For this review, take the finished solid that the model builds, in its own axes (mm). Coordinates: 2 decimals unless noted, no trailing zeros. Write each loop counter-clockwise with the first axis right and the second up, starting at its lowest first coordinate (ties: lowest second). Pieces come first, ordered by that corner, then holes.
```python
from build123d import *

# Parameters (mm, degrees)
F0_W     = 170
F0_H     = 40
F1_DEPTH = 1000
F3_DEPTH = 170.001
F4_SIZE2 = 25
F4_SIZE  = 25
F5_SIZE2 = 25
F5_SIZE  = 25
F6_R     = 4


with BuildPart() as f1:
    # F0 (on Top) → F1 (new body)
    with BuildSketch(Plane.XY):
        Rectangle(F0_W, F0_H)
    extrude(amount=F1_DEPTH)

    # F2 (on face) → F3 (cut, through all)
    with BuildSketch(Plane.YZ.offset(85)):
        Polygon((-20, 0), (18, 0), (-20, 38), align=None)
        Polygon((-20, 962), (18, 1000), (-20, 1000), align=None)
    extrude(amount=-F3_DEPTH, mode=Mode.SUBTRACT)

    # F4
    f4_edges = [f1.edges().sort_by_distance(p)[0] for p in [
        (85, -20, 500),
    ]]
    chamfer(f4_edges, length=F4_SIZE, length2=F4_SIZE2)

    # F5
    f5_edges = [f1.edges().sort_by_distance(p)[0] for p in [
        (-85, -20, 500),
    ]]
    chamfer(f5_edges, length=F5_SIZE, length2=F5_SIZE2)

    # F6
    f6_edges = [f1.edges().sort_by_distance(p)[0] for p in [
        (60, -20, 500),
        (0, -20, 38),
        (72.5, -7.5, 25.5),
        (85, 11.5, 6.5),
        (85, 5, 500),
        (-85, 11.5, 6.5),
        (-72.5, -7.5, 25.5),
        (-60, -20, 500),
        (72.5, -7.5, 974.5),
        (0, -20, 962),
        (85, 11.5, 993.5),
        (-72.5, -7.5, 974.5),
        (-85, 11.5, 993.5),
        (-85, 5, 500),
    ]]
    fillet(f6_edges, radius=F6_R)


solid = f1.part
```
Q1. Add section B-B (z = 673). State the section outline as (x, y) points, then the cut area to 3 significant figures.
Ans:
outline: (-85, 6.66) arc R4 ccw to (-83.83, 3.83) - (-61.17, -18.83) arc R4 ccw to (-58.34, -20) - (58.34, -20) arc R4 ccw to (61.17, -18.83) - (83.83, 3.83) arc R4 ccw to (85, 6.66) - (85, 20) - (-85, 20) - close
area: 6,170 mm2
Q2. Clearance check with flat-ended pins moving along their axes: pin 1 Ø1 at (y, z) = (-12, 132) entering from +X; pin 2 Ø1 at (y, z) = (0, 522.5) entering from -X; pin 3 Ø10 at (y, z) = (-13, 115.5) entering from +X. State where each tip first meets the part, or that it passes through.
Ans:
pin 1: stops at x = 68.5
pin 2: stops at x = -80.5
pin 3: stops at x = 72
Q3. Add section A-A (x = 0). State the section outline as (y, z) points, then the cut area to 3 significant figures.
Ans:
outline: (-20, 39.66) arc R4 ccw to (-18.83, 36.83) - (18, 0) - (20, 0) - (20, 1000) - (18, 1000) - (-18.83, 963.17) arc R4 ccw to (-20, 960.34) - close
area: 38,600 mm2
Q4. For probe 1 along X at (y, z) = (-18, 635.5); probe 2 along Z at (x, y) = (65.5, -7.5); probe 3 along X at (y, z) = (-13, 371.5), list the stretches that pass through material, from the lowest coordinate up.
Ans:
probe 1: x = -62 to 62
probe 2: z = 25.5 to 974.5
probe 3: x = -67 to 67
